For this review, take the finished solid that the model builds, in its own axes (mm). A direction names the side the tool comes from. Round coordinates to 2 decimals unless told otherwise and drop trailing zeros. Order: outer loops, then holes, each group sorted by start corner. A loop starts at its lowest first (then second) coordinate and runs counter-clockwise, first axis right, second up.
from build123d import *

# Parameters (mm, degrees)
SKETCH1_R             = 3
SKETCH1_R_2           = 1.55
BOSS_EXTRUDE1_DEPTH   = 3.5
BOSS_EXTRUDE1_2_DEPTH = 3.5
BOSS_EXTRUDE1_3_DEPTH = 3.5
BOSS_EXTRUDE1_4_DEPTH = 3.5
SKETCH2_R             = 3
SKETCH2_R_2           = 1.55
BOSS_EXTRUDE2_DEPTH   = 2.5
SKETCH3_W             = 6
SKETCH3_H             = 6
BOSS_EXTRUDE3_DEPTH   = 5
SKETCH4_W             = 6
SKETCH4_H             = 15
BOSS_EXTRUDE4_DEPTH   = 2.5
SKETCH5_W             = 4
SKETCH5_H             = 6
BOSS_EXTRUDE5_DEPTH   = 21.9
SKETCH6_W             = 6.7
SKETCH6_H             = 15
BOSS_EXTRUDE6_DEPTH   = 2.5
SKETCH7_R             = 1.55
SKETCH7_R_2           = 1.1
BOSS_EXTRUDE7_DEPTH   = 6


with BuildPart() as part:
    # Sketch1 → Boss-Extrude1 (new body)
    with BuildSketch(Plane(origin=(0, 0, 0), x_dir=(0, 0, -1), z_dir=(1, 0, 0))):
        with Locations((-47.5, 16.5)):
            Circle(SKETCH1_R)
        with Locations((-47.5, 16.5)):
            Circle(SKETCH1_R_2, mode=Mode.SUBTRACT)
    extrude(amount=BOSS_EXTRUDE1_DEPTH)



with BuildPart() as body_2:
    # Sketch1 → Boss-Extrude1 2 (new body)
    with BuildSketch(Plane(origin=(0, 0, 0), x_dir=(0, 0, -1), z_dir=(1, 0, 0))):
        with Locations((-47.5, -16.5)):
            Circle(SKETCH1_R)
        with Locations((-47.5, -16.5)):
            Circle(SKETCH1_R_2, mode=Mode.SUBTRACT)
    extrude(amount=BOSS_EXTRUDE1_2_DEPTH)


with BuildPart() as body_3:
    # Sketch1 → Boss-Extrude1 3 (new body)
    with BuildSketch(Plane(origin=(0, 0, 0), x_dir=(0, 0, -1), z_dir=(1, 0, 0))):
        with Locations((47.5, -16.5)):
            Circle(SKETCH1_R)
        with Locations((47.5, -16.5)):
            Circle(SKETCH1_R_2, mode=Mode.SUBTRACT)
    extrude(amount=BOSS_EXTRUDE1_3_DEPTH)


with BuildPart() as body_4:
    # Sketch1 → Boss-Extrude1 4 (new body)
    with BuildSketch(Plane(origin=(0, 0, 0), x_dir=(0, 0, -1), z_dir=(1, 0, 0))):
        with Locations((47.5, 16.5)):
            Circle(SKETCH1_R)
        with Locations((47.5, 16.5)):
            Circle(SKETCH1_R_2, mode=Mode.SUBTRACT)
    extrude(amount=BOSS_EXTRUDE1_4_DEPTH)


with BuildPart() as part_1:
    add(part.part)

    add(body_2.part)  # Boss-Extrude2 merges body 2

    add(body_3.part)  # Boss-Extrude2 merges body 3

    add(body_4.part)  # Boss-Extrude2 merges body 4
    # Sketch2 → Boss-Extrude2 (add)
    # profile 1 of 12: a face of its own
    with BuildSketch(Plane(origin=(3.5, 0, 0), x_dir=(0, 0, -1), z_dir=(1, 0, 0))):
        with BuildLine():
            Line((47.5, 19.5), (-47.5, 19.5))
            ThreePointArc((-47.5, 19.5), (-45.378679656, 18.621320344), (-44.5, 16.5))
            Line((-44.5, 16.5), (-44.5, 13.5))
            Line((-44.5, 13.5), (44.5, 13.5))
            Line((44.5, 13.5), (44.5, 16.5))
            ThreePointArc((44.5, 16.5), (45.378679656, 18.621320344), (47.5, 19.5))
        make_face()
    # profile 2 of 12: a face of its own
    with BuildSketch(Plane(origin=(3.5, 0, 0), x_dir=(0, 0, -1), z_dir=(1, 0, 0))):
        with Locations(Location((-47.5, 16.5, 0), (0, 0, 180))):
            Circle(SKETCH2_R)
        with Locations((-47.5, 16.5)):
            Circle(SKETCH2_R_2, mode=Mode.SUBTRACT)
    # profile 3 of 12: a face of its own
    with BuildSketch(Plane(origin=(3.5, 0, 0), x_dir=(0, 0, -1), z_dir=(1, 0, 0))):
        with BuildLine():
            Line((-44.5, 13.5), (-44.5, 16.5))
            ThreePointArc((-44.5, 16.5), (-45.378679656, 14.378679656), (-47.5, 13.5))
            Line((-47.5, 13.5), (-44.5, 13.5))
        make_face()
    # profile 4 of 12: a face of its own
    with BuildSketch(Plane(origin=(3.5, 0, 0), x_dir=(0, 0, -1), z_dir=(1, 0, 0))):
        with BuildLine():
            ThreePointArc((-47.5, 13.5), (-49.621320344, 14.378679656), (-50.5, 16.5))
            Line((-50.5, 16.5), (-50.5, -16.5))
            ThreePointArc((-50.5, -16.5), (-49.621320344, -14.378679656), (-47.5, -13.5))
            Line((-47.5, -13.5), (-44.5, -13.5))
            Line((-44.5, -13.5), (-44.5, 13.5))
            Line((-44.5, 13.5), (-47.5, 13.5))
        make_face()
    # profile 5 of 12: a face of its own
    with BuildSketch(Plane(origin=(3.5, 0, 0), x_dir=(0, 0, -1), z_dir=(1, 0, 0))):
        with BuildLine():
            Line((-44.5, -16.5), (-44.5, -13.5))
            Line((-44.5, -13.5), (-47.5, -13.5))
            ThreePointArc((-47.5, -13.5), (-45.378679656, -14.378679656), (-44.5, -16.5))
        make_face()
    # profile 6 of 12: a face of its own
    with BuildSketch(Plane(origin=(3.5, 0, 0), x_dir=(0, 0, -1), z_dir=(1, 0, 0))):
        with BuildLine():
            Line((44.5, -13.5), (-44.5, -13.5))
            Line((-44.5, -13.5), (-44.5, -16.5))
            ThreePointArc((-44.5, -16.5), (-45.378679656, -18.621320344), (-47.5, -19.5))
            Line((-47.5, -19.5), (47.5, -19.5))
            ThreePointArc((47.5, -19.5), (45.378679656, -18.621320344), (44.5, -16.5))
            Line((44.5, -16.5), (44.5, -13.5))
        make_face()
    # profile 7 of 12: a face of its own
    with BuildSketch(Plane(origin=(3.5, 0, 0), x_dir=(0, 0, -1), z_dir=(1, 0, 0))):
        with Locations(Location((-47.5, -16.5, 0), (0, 0, 180))):
            Circle(SKETCH2_R)
        with Locations((-47.5, -16.5)):
            Circle(SKETCH2_R_2, mode=Mode.SUBTRACT)
    # profile 8 of 12: a face of its own
    with BuildSketch(Plane(origin=(3.5, 0, 0), x_dir=(0, 0, -1), z_dir=(1, 0, 0))):
        with BuildLine():
            Line((50.5, -16.5), (50.5, 16.5))
            ThreePointArc((50.5, 16.5), (49.621320344, 14.378679656), (47.5, 13.5))
            Line((47.5, 13.5), (44.5, 13.5))
            Line((44.5, 13.5), (44.5, -13.5))
            Line((44.5, -13.5), (47.5, -13.5))
            ThreePointArc((47.5, -13.5), (49.621320344, -14.378679656), (50.5, -16.5))
        make_face()
    # profile 9 of 12: a face of its own
    with BuildSketch(Plane(origin=(3.5, 0, 0), x_dir=(0, 0, -1), z_dir=(1, 0, 0))):
        with BuildLine():
            ThreePointArc((44.5, -16.5), (45.378679656, -14.378679656), (47.5, -13.5))
            Line((47.5, -13.5), (44.5, -13.5))
            Line((44.5, -13.5), (44.5, -16.5))
        make_face()
    # profile 10 of 12: a face of its own
    with BuildSketch(Plane(origin=(3.5, 0, 0), x_dir=(0, 0, -1), z_dir=(1, 0, 0))):
        with Locations((47.5, -16.5)):
            Circle(SKETCH2_R)
        with Locations((47.5, -16.5)):
            Circle(SKETCH2_R_2, mode=Mode.SUBTRACT)
    # profile 11 of 12: a face of its own
    with BuildSketch(Plane(origin=(3.5, 0, 0), x_dir=(0, 0, -1), z_dir=(1, 0, 0))):
        with BuildLine():
            ThreePointArc((47.5, 13.5), (45.378679656, 14.378679656), (44.5, 16.5))
            Line((44.5, 16.5), (44.5, 13.5))
            Line((44.5, 13.5), (47.5, 13.5))
        make_face()
    # profile 12 of 12: a face of its own
    with BuildSketch(Plane(origin=(3.5, 0, 0), x_dir=(0, 0, -1), z_dir=(1, 0, 0))):
        with Locations((47.5, 16.5)):
            Circle(SKETCH2_R)
        with Locations((47.5, 16.5)):
            Circle(SKETCH2_R_2, mode=Mode.SUBTRACT)
    extrude(amount=BOSS_EXTRUDE2_DEPTH)

    # Sketch3 → Boss-Extrude3 (add)
    with BuildSketch(Plane(origin=(6, 0, 0), x_dir=(0, 0, -1), z_dir=(1, 0, 0))):
        with Locations((47.5, -10.5)):
            Rectangle(SKETCH3_W, SKETCH3_H)
        with Locations((-47.5, -10.5)):
            Rectangle(SKETCH3_W, SKETCH3_H)
    extrude(amount=BOSS_EXTRUDE3_DEPTH)

    # Sketch4 → Boss-Extrude4 (add)
    with BuildSketch(Plane(origin=(11, 0, 0), x_dir=(0, 0, -1), z_dir=(1, 0, 0))):
        with Locations((47.5, -15)):
            Rectangle(SKETCH4_W, SKETCH4_H)
    extrude(amount=BOSS_EXTRUDE4_DEPTH)

    # Sketch5 → Boss-Extrude5 (add)
    with BuildSketch(Plane.XY.offset(50.5)):
        with Locations((9, -10.5)):
            Rectangle(SKETCH5_W, SKETCH5_H)
    extrude(amount=BOSS_EXTRUDE5_DEPTH)

    # Sketch6 → Boss-Extrude6 (add)
    with BuildSketch(Plane(origin=(11, 0, 0), x_dir=(0, 0, -1), z_dir=(1, 0, 0))):
        with Locations((-69.05, -15)):
            Rectangle(SKETCH6_W, SKETCH6_H)
    extrude(amount=BOSS_EXTRUDE6_DEPTH)


with BuildPart() as body_2_2:
    # Split1: the piece on the far side of the plane
    add(part_1.part)
    split(bisect_by=Plane(origin=(6, 0, 0), x_dir=(0, 0, 1), z_dir=(1, 0, 0)), keep=Keep.BOTTOM)

    # Sketch7 → Boss-Extrude7 (add)
    with BuildSketch(Plane.ZY):
        with Locations((47.5, -16.5)):
            Circle(SKETCH7_R)
        with Locations((47.5, -16.5)):
            Circle(SKETCH7_R_2, mode=Mode.SUBTRACT)
    extrude(amount=-BOSS_EXTRUDE7_DEPTH)


with BuildPart() as part_2:
    add(part_1.part)

    # Split1
    split(bisect_by=Plane(origin=(6, 0, 0), x_dir=(0, 0, 1), z_dir=(1, 0, 0)), keep=Keep.TOP)


solid = body_2_2.part
(1) Add section C-C on x = 4.6. Give the boundary of the cut face in (y, z).
(2) Wall thickness on L1, parallel to Y at x = 1.3, z = -47.5; L2, parallel to Z at x = 4.75, y = 10.5; L3, parallel to Y at x = 3.85, z = 47.5: over which ranges is each line inside the solid? List them lowest first.
(3) Tool access review of faces 1 (the face through (5, 0, -50.5)), 2 (the face through (3.5, -14, -4)), 3 (the face through (5, -13.5, -1)): name each direction out of +Z, -Z, +X, -X, +Y, -Y from which nothing blocks a thin tool from reaching the whole face with its end or side.
(4) Add section B-B on z = -18. Give the boundary of the cut face in (x, y), plus the area to 3 significant figures.
(5) Add section A-A on y = -1.5. Give the boundary of the cut face in (x, z).
Here are the results:
1. outline: (-19.5, -47.5) arc R3 ccw to (-16.5, -50.5) - (16.5, -50.5) arc R3 ccw to (19.5, -47.5) - (19.5, 47.5) arc R3 ccw to (16.5, 50.5) - (-16.5, 50.5) arc R3 ccw to (-19.5, 47.5) - close; hole circle Ø3.1 at (-16.5, -47.5); hole circle Ø2.2 at (-16.5, 47.5); hole (-13.5, -44.5) - (13.5, -44.5) - (13.5, 44.5) - (-13.5, 44.5) - close; hole circle Ø3.1 at (16.5, -47.5); hole circle Ø3.1 at (16.5, 47.5)
2. L1: y = -19.5 to -18.05, -14.95 to -13.5, 13.5 to 14.95, 18.05 to 19.5
2. L2: z = -50.5 to -44.5, 44.5 to 50.5
2. L3: y = -19.5 to -17.6, -15.4 to 14.95, 18.05 to 19.5
3. face 1: -Z, +X, -X, +Y, -Y
3. face 2: -X
3. face 3: +X, -X
4. outline: (3.5, -19.5) - (6, -19.5) - (6, -13.5) - (3.5, -13.5) - close; (3.5, 13.5) - (6, 13.5) - (6, 19.5) - (3.5, 19.5) - close
4. area: 30.0 mm2
5. outline: (3.5, -50.5) - (6, -50.5) - (6, -44.5) - (3.5, -44.5) - close; (3.5, 44.5) - (6, 44.5) - (6, 50.5) - (3.5, 50.5) - close
